from build123d import *

# Parameters (mm, degrees)
F0_W     = 34.33
F0_H     = 17.8
F1_DEPTH = 1.25
F2_W     = 31.5
F2_H     = 14.8
F3_DEPTH = 4.18
F4_W     = 7.7
F4_H     = 3
F5_DEPTH = 2.36
F6_W     = 5.033333
F6_H     = 2.8
F7_DEPTH = 6.33


with BuildPart() as f1:
    # F0 (on Top) → F1 (new body)
    with BuildSketch(Plane.XY):
        with Locations((17.165, 8.9)):
            Rectangle(F0_W, F0_H)
    extrude(amount=F1_DEPTH)

    # F2 (on face) → F3 (join)
    with BuildSketch(Plane.XY.offset(1.25)):
        with Locations((15.75, 8.9)):
            Rectangle(F2_W, F2_H)
    extrude(amount=F3_DEPTH)

    # F4 (on face) → F5 (join)
    with BuildSketch(Plane(origin=(0, 0, 0), x_dir=(0, -1, 0), z_dir=(-1, 0, 0))):
        with Locations((-11.59, 0.15)):
            Rectangle(F4_W, F4_H)
    extrude(amount=F5_DEPTH)

    # F6 (on face) → F7 (join)
    with BuildSketch(Plane(origin=(-2.36, 0, 0), x_dir=(0, -1, 0), z_dir=(-1, 0, 0))):
        with Locations((-12.823334, 0.15)):
            Rectangle(F6_W, F6_H)
    extrude(amount=F7_DEPTH)


solid = f1.part
The model under review builds one solid part; all positions refer to its coordinate system, in mm. A direction names the side the tool comes from. Coordinates: 2 decimals unless noted, no trailing zeros. Write each loop counter-clockwise with the first axis right and the second up, starting at its lowest first coordinate (ties: lowest second). Pieces come first, ordered by that corner, then holes. Notation, with made-up numbers: M 61,58.25 L 118,58.25 A12 cw 118,65.25 Z; hole C 49,-8 d8. An arc over 180 degrees is marked long. Put each result on its own line as item: value.
1) Add section B-B on x = 2. Give the boundary of the cut face in (y, z), then the cut area to 3 significant figures.
Computed:
outline: M 0,0 L 17.8,0 L 17.8,1.25 L 16.3,1.25 L 16.3,5.43 L 1.5,5.43 L 1.5,1.25 L 0,1.25 Z
area: 84.1 mm2
2) For faces 1 (the flat face through (0, 12, -1)), 2 (the flat face through (-5, 15.34, 0)), 3 (the flat face through (-5, 13, -1.25)), list the 3-axis set-ups (+Z, -Z, +X, -X, +Y, -Y) from which the entire face can be reached by the end or side of a thin tool; tool diameter is ignored.
Computed:
face 1: -Z, +X, +Y, -Y
face 2: +Z, -Z, -X, +Y
face 3: -Z, -X, +Y, -Y
3) Clearance check with flat-ended pins moving along their axes: pin 1 Ø1.5 at (x, y) = (22, 3.5) entering from -Z; pin 2 Ø4 at (x, y) = (-6.5, 14) entering from -Z; pin 3 Ø1.6 at (y, z) = (8.5, 4) entering from -X. State where each tip first meets the part, or that it passes through.
Computed:
pin 1: stops at z = 0
pin 2: stops at z = -1.25
pin 3: stops at x = 0
4) Add section C-C on y = 9.75. Give the boundary of the cut face in (x, z), then the cut area to 3 significant figures.
Computed:
outline: M -2.36,-1.35 L 0,-1.35 L 0,0 L 34.33,0 L 34.33,1.25 L 31.5,1.25 L 31.5,5.43 L 0,5.43 L 0,1.65 L -2.36,1.65 Z
area: 182 mm2
5) Wall thickness on probe 1 along Y at (x, z) = (22.5, 3.5); probe 2 along X at (y, z) = (15.5, 3.5); probe 3 along Y at (x, z) = (-3, 0): over which ranges is each line inside the solid? List them lowest first. Write a range as [from, to].
Computed:
probe 1: y = [1.5, 16.3]
probe 2: x = [0, 31.5]
probe 3: y = [10.31, 15.34]
6) Add section A-A on z = -0.75. Give the boundary of the cut face in (x, y).
Computed:
outline: M -8.69,10.31 L -2.36,10.31 L -2.36,7.74 L 0,7.74 L 0,15.44 L -2.36,15.44 L -2.36,15.34 L -8.69,15.34 Z
7) Add section D-D on y = 13.75. Give the boundary of the cut face in (x, z).
Computed:
outline: M -8.69,-1.25 L -2.36,-1.25 L -2.36,-1.35 L 0,-1.35 L 0,0 L 34.33,0 L 34.33,1.25 L 31.5,1.25 L 31.5,5.43 L 0,5.43 L 0,1.65 L -2.36,1.65 L -2.36,1.55 L -8.69,1.55 Z
